Part print with two shaded views. Sizes in mm from the minimum x, y, z corner. A direction names the side the tool comes from. Round coordinates to 2 decimals unless told otherwise and drop trailing zeros. Loops run counter-clockwise (first coordinate to the right, second up) from the corner with the lowest first, then second, coordinate; pieces in that order, holes last. Notation, with made-up numbers: M 57,55 L 110,55 A9 cw 110,61 Z; hole C 57.25,83.5 d9. An arc over 180 degrees is marked long. Use a Markdown table: item, result. Add a question column.
Item 1: Tool access for the marked faces 1 and 2: list every direction of +Z, -Z, +X, -X, +Y, -Y with a clear straight run to the whole face (end or side of a thin tool).
Item 2: Saw through at D-D on x = 4. Write the cut outline in (y, z), then the cut area to 3 significant figures.
Item 3: Saw through at C-C on z = 14. Write the cut outline in (x, y), then the cut area to 3 significant figures.
Item 4: Wall check: L1, parallel to Z at x = 4, y = 18.5; L2, parallel to Z at x = 25.5, y = 15; L3, parallel to X at y = 20.5, z = 24. Give the ranges that are in metal, low to high. Write a range as from..to.
Item 5: Saw through at A-A on x = 20. Write the cut outline in (y, z) (3 decimals).
Item 6: Pin check, flat tips, straight feed: P1, Ø10, axis at x = 9, y = 13.5, coming from the -Z side; P2, Ø1, axis at x = 34.5, y = 31, coming from the +Z side; P3, Ø3, axis at y = 10, z = 32.5, coming from the -X side; P4, Ø8, axis at y = 26, z = 20, coming from the +X side. Stop position of each tip, or through.
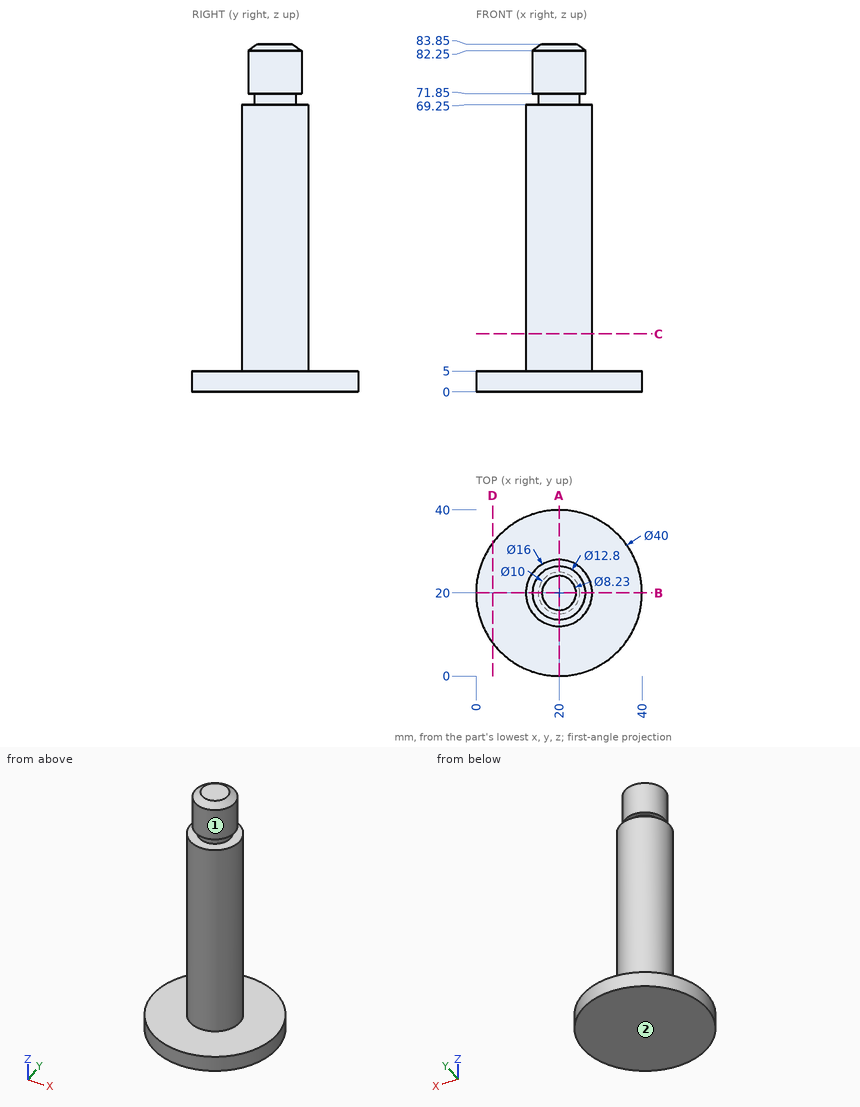
Entries:
| question | item | result |
|---|---|---|
| 1 | face 1 | +Z |
| 1 | face 2 | -Z, +X, -X, +Y, -Y |
| 2 | outline | M 8,0 L 32,0 L 32,5 L 8,5 Z |
| 2 | area | 120 mm2 |
| 3 | outline | C 20,20 d16 |
| 3 | area | 201 mm2 |
| 4 | L1 | 0..5 |
| 4 | L2 | 0..69.25 |
| 4 | L3 | 12.02..27.98 |
| 5 | outline | M 0,0 L 40,0 L 40,5 L 28,5 L 28,69.25 L 25,69.25 L 25,71.85 L 26.4,71.85 L 26.4,82.25 L 24.115,83.85 L 15.885,83.85 L 13.6,82.25 L 13.6,71.85 L 15,71.85 L 15,69.25 L 12,69.25 L 12,5 L 0,5 Z |
| 6 | P1 | z = 0 |
| 6 | P2 | z = 5 |
| 6 | P3 | through |
| 6 | P4 | x = 27.75 |
